```python
from build123d import *

# Parameters (mm, degrees)
EXTRUDE_DEPTH     = 5
EXTRUDE001_DEPTH  = 5
BOX054_W          = 128
BOX054_H          = 10
BOX054_DEPTH      = 5
BOX055_W          = 128
BOX055_H          = 10
BOX055_DEPTH      = 5
CYLINDER160_R     = 1.7
CYLINDER160_DEPTH = 4
CYLINDER161_R     = 1.7
CYLINDER161_DEPTH = 4
CYLINDER147_R     = 7
CYLINDER147_DEPTH = 4
BOX061_W          = 4
BOX061_H          = 38
BOX061_DEPTH      = 18
CHAMFER005_SIZE   = 1
CHAMFER006_SIZE   = 1
CYLINDER114_R     = 4.1
CYLINDER114_DEPTH = 10
TUBE_R            = 6
TUBE_R_2          = 4.5
TUBE_DEPTH        = 6
BOX053_W          = 86
BOX053_H          = 38
BOX053_DEPTH      = 5
CHAMFER007_SIZE   = 3


with BuildPart() as extrude_body:
    # Sketch → Extrude (new body)
    with BuildSketch(Plane.XZ):
        Polygon((132.822781, 16.830847), (111.859555, 33.003719), (91.859555, 33.003719), (91.859555, 28.003719), (107.162236, 16.830847), align=None)
    extrude(amount=EXTRUDE_DEPTH)


with BuildPart() as extrude_body_1:
    # Extrude placement: moved
    add(extrude_body.part.moved(Location((0, 4, 0))))


with BuildPart() as extrude001:
    # Sketch → Extrude001 (new body)
    with BuildSketch(Plane.XZ):
        Polygon((132.822781, 16.830847), (111.859555, 33.003719), (91.859555, 33.003719), (91.859555, 28.003719), (107.162236, 16.830847), align=None)
    extrude(amount=EXTRUDE001_DEPTH)


with BuildPart() as extrude001_1:
    # Extrude001 placement: moved
    add(extrude001.part.moved(Location((0, -39, 0))))


with BuildPart() as cube054:
    # Box054 → Box054 (new body)
    with BuildSketch(Plane(origin=(107, -39, 7), x_dir=(1, 0, 0), z_dir=(0, -1, 0))):
        with Locations((64, 5)):
            Rectangle(BOX054_W, BOX054_H)
    extrude(amount=BOX054_DEPTH)


with BuildPart() as cube055:
    # Box055 → Box055 (new body)
    with BuildSketch(Plane(origin=(107, 4, 7), x_dir=(1, 0, 0), z_dir=(0, -1, 0))):
        with Locations((64, 5)):
            Rectangle(BOX055_W, BOX055_H)
    extrude(amount=BOX055_DEPTH)


with BuildPart() as cylinder160:
    # Cylinder160 → Cylinder160 (new body)
    with BuildSketch(Plane(origin=(126, 0, 12), x_dir=(0, 0, 1), z_dir=(-1, 0, 0))):
        Circle(CYLINDER160_R)
    extrude(amount=CYLINDER160_DEPTH)


with BuildPart() as fusion:
    # Cylinder161 → Cylinder161 (new body)
    with BuildSketch(Plane(origin=(126, 25, 12), x_dir=(0, 0, 1), z_dir=(-1, 0, 0))):
        Circle(CYLINDER161_R)
    extrude(amount=CYLINDER161_DEPTH)

    # Fusion: union Cylinder160
    add(cylinder160.part)


with BuildPart() as fusion_1:
    # Fusion placement: moved
    add(fusion.part.moved(Location((0, -32.5, 0))))


with BuildPart() as cylinder147:
    # Cylinder147 → Cylinder147 (new body)
    with BuildSketch(Plane(origin=(122, -20, 12), x_dir=(0, 0, -1), z_dir=(1, 0, 0))):
        Circle(CYLINDER147_R)
    extrude(amount=CYLINDER147_DEPTH)


with BuildPart() as chamfer006:
    # Box061 → Box061 (new body)
    with BuildSketch(Plane(origin=(122, -39, 3), x_dir=(1, 0, 0), z_dir=(0, 0, 1))):
        with Locations((2, 19)):
            Rectangle(BOX061_W, BOX061_H)
    extrude(amount=BOX061_DEPTH)

    # Cut085: cut Cylinder147
    add(cylinder147.part, mode=Mode.SUBTRACT)

    # Cut088: cut Fusion
    add(fusion_1.part, mode=Mode.SUBTRACT)

    # Chamfer005
    chamfer005_edges = [chamfer006.edges().sort_by_distance(p)[0] for p in [
        (122, -7.5, 10.3),
        (122, -20, 19),
    ]]
    chamfer(chamfer005_edges, length=CHAMFER005_SIZE)

    # Chamfer006
    chamfer006_edges = [chamfer006.edges().sort_by_distance(p)[0] for p in [
        (126, -20, 19),
    ]]
    chamfer(chamfer006_edges, length=CHAMFER006_SIZE)


with BuildPart() as cylinder114:
    # Cylinder114 → Cylinder114 (new body)
    with BuildSketch(Plane(origin=(37, -20, 21), x_dir=(1, 0, 0), z_dir=(0, 0, 1))):
        Circle(CYLINDER114_R)
    extrude(amount=CYLINDER114_DEPTH)


with BuildPart() as tube:
    # Tube → Tube (new body)
    with BuildSketch(Plane(origin=(37, -20, 21), x_dir=(1, 0, 0), z_dir=(0, 0, 1))):
        Circle(TUBE_R)
        Circle(TUBE_R_2, mode=Mode.SUBTRACT)
    extrude(amount=TUBE_DEPTH)


with BuildPart() as chamfer007:
    # Box053 → Box053 (new body)
    with BuildSketch(Plane(origin=(26, -39, 22), x_dir=(1, 0, 0), z_dir=(0, 0, 1))):
        with Locations((43, 19)):
            Rectangle(BOX053_W, BOX053_H)
    extrude(amount=BOX053_DEPTH)

    # Fusion092: union Tube
    add(tube.part)

    # Cut073: cut Cylinder114
    add(cylinder114.part, mode=Mode.SUBTRACT)


with BuildPart() as chamfer007_1:
    # Cut073 placement: moved
    add(chamfer007.part.moved(Location((0, 0, 6))))

    # Fusion112: union Extrude body, Extrude001, Cube054, Cube055, Chamfer006
    add(extrude_body_1.part)
    add(extrude001_1.part)
    add(cube054.part)
    add(cube055.part)
    add(chamfer006.part)

    # Chamfer007
    chamfer007_edges = [chamfer007_1.edges().sort_by_distance(p)[0] for p in [
        (124, -1, 3),
        (124, -39, 3),
    ]]
    chamfer(chamfer007_edges, length=CHAMFER007_SIZE)


solid = chamfer007_1.part
```
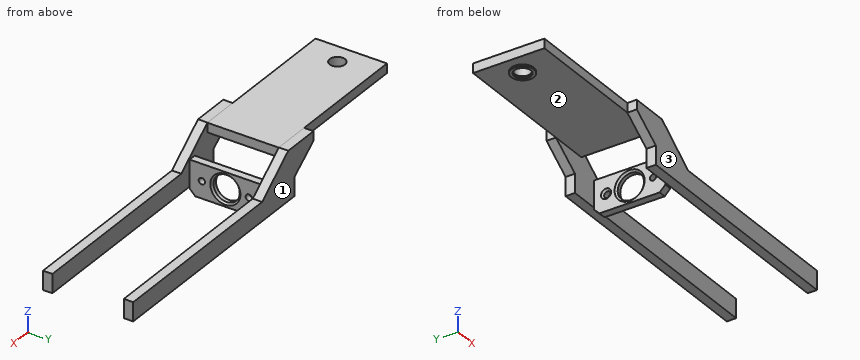
Model file for the job. Use its own axes, mm. Face numbers are marked on the shaded views. Give positions to 0.01 mm unless a question says otherwise; leave off trailing zeros. Loops run counter-clockwise (first coordinate to the right, second up) from the corner with the lowest first, then second, coordinate; pieces in that order, holes last. Notation, with made-up numbers: (33, 28.25) -> (83, 28.25) arc R20 ccw to (83, 65.25) -> close; hole circle Ø10 at (32, 5). An arc over 180 degrees is marked (long way). Use CSV: the item, a comma, the result in double quotes. Start each with the question number.
1) Wall check: line 1 (Y direction, x = 123, z = 12); line 2 (X direction, y = -20, z = 27.3); line 3 (Y direction, x = 102.5, z = 24). Give the ranges that are in metal, low to high.
2) Flat gauge pins, fed straight in: pin 1 Ø10.5 at (x, y) = (37, -20) entering from +Z; pin 2 Ø2 at (x, y) = (125, -18.5) entering from +Z; pin 3 Ø19 at (x, y) = (63.5, -10.5) entering from -Z. Where does each tip first touch, or does it go through?
3) Mould opens along Y. For the marked faces 1, 2 and 3 say: released by +Y, released by -Y, zero draft, split by the parting line, or undercut.
4) Slice it at C-C on z = 23.5. Give the cut face in (x, y), plus the area to 3 significant figures.
5) Slice it at B-B on x = 37. Give the cut face in (y, z).
6) Slice it at A-A on y = -20. Give the cut face in (x, z).
Computed values:
1,line 1,"y = -44 to -34.2, -30.8 to -27, -13 to -9.2, -5.8 to 4"
1,line 2,"x = 31 to 32.5, 41.5 to 43"
1,line 3,"y = -44 to -39, -1 to 4"
2,pin 1,"stops at z = 33"
2,pin 2,"stops at z = 21"
2,pin 3,"stops at z = 28"
3,face 1,"released by +Y"
3,face 2,"undercut"
3,face 3,"released by -Y"
4,outline,"(98.03, -44) -> (124.18, -44) -> (124.18, -39) -> (98.03, -39) -> close; (98.03, -1) -> (124.18, -1) -> (124.18, 4) -> (98.03, 4) -> close"
4,area,"262 mm^2"
5,outline,"(-39, 28) -> (-26, 28) -> (-26, 27) -> (-24.5, 27) -> (-24.5, 28) -> (-24.1, 28) -> (-24.1, 33) -> (-39, 33) -> close; (-15.9, 28) -> (-15.5, 28) -> (-15.5, 27) -> (-14, 27) -> (-14, 28) -> (-1, 28) -> (-1, 33) -> (-15.9, 33) -> close"
6,outline,"(26, 28) -> (31, 28) -> (31, 27) -> (32.5, 27) -> (32.5, 28) -> (32.9, 28) -> (32.9, 33) -> (26, 33) -> close; (41.1, 28) -> (41.5, 28) -> (41.5, 27) -> (43, 27) -> (43, 28) -> (112, 28) -> (112, 33) -> (41.1, 33) -> close; (122, 3) -> (126, 3) -> (126, 4) -> (125, 5) -> (123, 5) -> (122, 4) -> close; (122, 20) -> (123, 19) -> (125, 19) -> (126, 20) -> (126, 21) -> (122, 21) -> close"
